Source: CAD feature listing. Evaluate the final solid. Frame: model axes, mm. A direction names the side the tool comes from. Round coordinates to 2 decimals unless told otherwise and drop trailing zeros. Loops run counter-clockwise (first coordinate to the right, second up) from the corner with the lowest first, then second, coordinate; pieces in that order, holes last. Notation, with made-up numbers: (82.5, 68) - (138.5, 68) arc R24 cw to (138.5, 89) - close; hole circle Ø7 at (26, 76). An arc over 180 degrees is marked (long way). One line per question, with ' | ' between items.
from build123d import *

# Parameters (mm, degrees)
F1_DEPTH       = 5
F2_D           = 3.3
F2_CBORE_D     = 6.5
F2_CBORE_DEPTH = 3


with BuildPart() as f1:
    # F0 (on Right) → F1 (new body)
    with BuildSketch(Plane.YZ):
        with BuildLine():
            Line((-21.4785121566, 4.7616715066), (-25.3836961851, 5.6274299624))
            ThreePointArc((-25.3836961851, 5.6274299624), (-18.3847763109, -18.3847763109), (5.6274299624, -25.3836961851))
            Line((5.6274299624, -25.3836961851), (4.7616715066, -21.4785121566))
            ThreePointArc((4.7616715066, -21.4785121566), (2.3950712467, -21.8692394409), (0, -22))
            ThreePointArc((0, -22), (-4.2919870844, -21.5772761689), (-8.419035512, -20.3253497152))
            ThreePointArc((-8.419035512, -20.3253497152), (-12.2225451264, -18.2923314707), (-15.5563491861, -15.5563491861))
            ThreePointArc((-15.5563491861, -15.5563491861), (-18.2923314707, -12.2225451264), (-20.3253497152, -8.419035512))
            ThreePointArc((-20.3253497152, -8.419035512), (-21.5772761689, -4.2919870844), (-22, 0))
            ThreePointArc((-22, 0), (-21.8692394409, 2.3950712467), (-21.4785121566, 4.7616715066))
        make_face()
        with BuildLine():
            Line((-17.5733281282, 3.8959130509), (-21.4785121566, 4.7616715066))
            ThreePointArc((-21.4785121566, 4.7616715066), (-21.8692394409, 2.3950712467), (-22, 0))
            ThreePointArc((-22, 0), (-21.5772761689, -4.2919870844), (-20.3253497152, -8.419035512))
            ThreePointArc((-20.3253497152, -8.419035512), (-18.2923314707, -12.2225451264), (-15.5563491861, -15.5563491861))
            ThreePointArc((-15.5563491861, -15.5563491861), (-12.2225451264, -18.2923314707), (-8.419035512, -20.3253497152))
            ThreePointArc((-8.419035512, -20.3253497152), (-4.2919870844, -21.5772761689), (0, -22))
            ThreePointArc((0, -22), (2.3950712467, -21.8692394409), (4.7616715066, -21.4785121566))
            Line((4.7616715066, -21.4785121566), (3.8959130509, -17.5733281282))
            ThreePointArc((3.8959130509, -17.5733281282), (-12.7279220614, -12.7279220614), (-17.5733281282, 3.8959130509))
        make_face()
        with BuildLine():
            Line((-3.9051840285, 0.8657584558), (-17.5733281282, 3.8959130509))
            ThreePointArc((-17.5733281282, 3.8959130509), (-12.7279220614, -12.7279220614), (3.8959130509, -17.5733281282))
            Line((3.8959130509, -17.5733281282), (0.8657584558, -3.9051840285))
            Line((0.8657584558, -3.9051840285), (0, 0))
            Line((0, 0), (-3.9051840285, 0.8657584558))
        make_face()
        with BuildLine():
            ThreePointArc((0.8657584558, -3.9051840285), (2.8284271247, 2.8284271247), (-3.9051840285, 0.8657584558))
            Line((-3.9051840285, 0.8657584558), (0, 0))
            Line((0, 0), (0.8657584558, -3.9051840285))
        make_face()
    extrude(amount=F1_DEPTH)

    # F2 (through all)
    with Locations(Plane(origin=(0, 0, 0), x_dir=(0, 1, 0), z_dir=(-1, 0, 0))):
        with Locations((-22, 0), (-20.3253497152, 8.419035512), (-15.5563491861, 15.5563491861), (-8.419035512, 20.3253497152), (0, 22), (0, 0)):
            CounterBoreHole(F2_D / 2, F2_CBORE_D / 2, F2_CBORE_DEPTH)


solid = f1.part
1. Contact query for a flat-ended pin moving along its axis: P1, Ø4, axis at y = -20.33, z = -8.42, coming from the -X side. Output: stop coordinate, or through.
Worked out:
P1: stops at x = 3
2. Access query for faces 4 (the flat face through (3, 1.4, 1.4)), 5 (the cylindrical face through (4.014, -9.306, -21.717)). Directions: +Z, -Z, +X, -X, +Y, -Y. A direction counts if a zero-diameter tool reaches every point of the face in a straight line with its end or side. Return the directions, or none.
Worked out:
face 4: -X | face 5: +X, -X
3. Mould query, pull axis Y, two halves, no side actions, for faces 1 (the cylindrical face through (4.014, 0.215, -23.636)), 2 (the cylindrical face through (4.01, -21.9, -8.91)), 3 (the flat face through (5, -10, -10)). Classes: released by +Y, released by -Y, zero draft, split by the parting line, or undercut.
Worked out:
face 1: undercut | face 2: undercut | face 3: zero draft
4. Section query D-D, the plane z = -22.5. Return loops of the section in (x, y), plus the area to 3 significant figures.
Worked out:
outline: (0, -13.03) - (5, -13.03) - (5, -1.57) - (3, -1.57) - (3, -3.21) - (0, -3.21) - (0, -6) - (3, -6) - (3, -10.83) - (0, -10.83) - close; (0, 3.21) - (3, 3.21) - (3, 1.57) - (5, 1.57) - (5, 4.99) - (0, 4.99) - close | area: 50.0 mm2
5. Material intervals for probe 1 along Z at (x, y) = (3.4, -21.5); probe 2 along Y at (x, z) = (1.2, -1.5); probe 3 along Z at (x, y) = (4.2, -20.5), sorted ascending.
Worked out:
probe 1: z = -14.62 to -9.58, -7.26 to -1.57, 1.57 to 4.77 | probe 2: y = -25.96 to -24.88, -19.12 to -2.88, 2.88 to 3.71 | probe 3: z = -15.99 to -10.06, -6.78 to -0.69, 0.69 to 4.54
6. Section query C-C, the plane y = -19.5. Return loops of the section in (x, z).
Worked out:
outline: (0, -17.2) - (5, -17.2) - (5, -9.85) - (3, -9.85) - (3, -11.56) - (0, -11.56) - close; (0, -5.28) - (3, -5.28) - (3, -6.99) - (5, -6.99) - (5, 4.32) - (0, 4.32) - (0, 2.08) - (3, 2.08) - (3, -2.08) - (0, -2.08) - close
7. Section query A-A, the plane y = 0. Return loops of the section in (x, z), plus the area to 3 significant figures.
Worked out:
outline: (0, -26) - (5, -26) - (5, -23.65) - (3, -23.65) - (3, -25.25) - (0, -25.25) - close; (0, -18.75) - (3, -18.75) - (3, -20.35) - (5, -20.35) - (5, -1.65) - (3, -1.65) - (3, -3.25) - (0, -3.25) - close; (0, 3.25) - (3, 3.25) - (3, 1.65) - (5, 1.65) - (5, 4) - (0, 4) - close | area: 97.8 mm2
